```python
from build123d import *

# Parameters (mm, degrees)
F1_DEPTH = 19.05
F2_R     = 5.08


with BuildPart() as f1:
    # F0 (on Front) → F1 (new body, symmetric)
    with BuildSketch(Plane.XZ):
        with BuildLine():
            ThreePointArc((-41.2102176428, -56.9380209093), (-42.7262869342, -63.8945167146), (-36.8305512568, -67.8859576583))
            Line((-36.8305512568, -67.8859576583), (56.6456316932, -67.8859576583))
            ThreePointArc((56.6456316932, -67.8859576583), (61.0217420398, -66.1372790157), (62.9876442917, -61.8543539524))
            Line((62.9876442917, -61.8543539524), (68.6381038561, 50.6949640107))
            ThreePointArc((68.6381038561, 50.6949640107), (65.1567213738, 60.0839772923), (55.954078659, 64.031756599))
            Line((55.954078659, 64.031756599), (0, 64.031756599))
            add(Edge.make_bspline(
                [(0, 64.031756599), (-13.8958169074, 92.772193382), (18.9529467347, 138.9305901021), (-24.5397146791, 107.536368072), (-61.751320227, 119.3237975012)],
                knots=[0, 0, 0, 0, 0.4861927134, 1, 1, 1, 1], degree=3))
            add(Edge.make_bspline(
                [(-41.2102176428, -56.9380209093), (-35.2492907521, -51.2600673928), (-10.330751513, -19.1265381914), (-62.4997914355, 44.8085571184), (-61.751320227, 119.3237975012)],
                knots=[0.1516920821, 0.1516920821, 0.1516920821, 0.1516920821, 0.3399970952, 1, 1, 1, 1], degree=3))
        make_face()
    extrude(amount=F1_DEPTH, both=True)

    # F2
    f2_edges = [f1.edges().sort_by_distance(p)[0] for p in [
        (-61.75132, -9.525, 119.323798),
        (-61.75132, 9.525, 119.323798),
    ]]
    fillet(f2_edges, radius=F2_R)


solid = f1.part
```
The model under review builds one solid part; all positions refer to its coordinate system, in mm. Round coordinates to 2 decimals unless told otherwise and drop trailing zeros. Write each loop counter-clockwise with the first axis right and the second up, starting at its lowest first coordinate (ties: lowest second). Pieces come first, ordered by that corner, then holes. Notation, with made-up numbers: (59, 83) - (83, 83) arc R19 cw to (83, 119) - close; hole circle Ø11 at (80, 4). An arc over 180 degrees is marked (long way). One line per question, with ' | ' between items.
Item 1: Add section A-A, the plane x = 4.5. Give the boundary of the cut face in (y, z).
Resolved:
outline: (-19.05, -67.89) - (19.05, -67.89) - (19.05, 64.03) - (-19.05, 64.03) - close
Item 2: For P1, Ø11.5, axis at x = 38, y = -4.5, coming from the +Z side; P2, Ø3, axis at y = 13.5, z = 75.5, coming from the -X side; P3, Ø5, axis at x = -47, y = -14, coming from the +Z side, all flat-tipped, find the tip position at first contact; note any pin that passes through.
Resolved:
P1: stops at z = 64.03 | P2: stops at x = -57.84 | P3: stops at z = 116.29
Item 3: To check wall thickness, follow probe 1 along Z at (x, y) = (35, -9); probe 2 along X at (y, z) = (-16, 70.5); probe 3 along Z at (x, y) = (-6, -4). State the ranges of each line that lie inside material, in increasing order.
Resolved:
probe 1: z = -67.89 to 64.03 | probe 2: x = -56.5 to -2.68 | probe 3: z = -67.89 to 119.34
Item 4: The part is to be moulded in two halves that separate along Z. For faces 1 (the face through (-42.765, -0.267, -63.796)), 2 (the face through (65.773, -0.267, -6.368)), 3 (the face through (3, 19.05, 13)), say which applies: pulls with the +Z half, pulls with the -Z half, needs draft (parallel to the pull), parting line crosses it, or undercut.
Resolved:
face 1: undercut | face 2: pulls with the -Z half | face 3: needs draft
